Autodesk Inventor part; units mm, degrees
ref_plane "YZ Plane" through (0, 0, 0) normal (1, 0, 0) x (0, 1, 0)
ref_plane "XZ Plane" through (0, 0, 0) normal (0, 1, 0) x (-1, 0, 0)
ref_plane "XY Plane" through (0, 0, 0) normal (0, 0, 1) x (1, 0, 0)
sketch "Sketch1" plane through (0, 0, 0) normal (0, 1, 0) x (-1, 0, 0)
  line L0 (0, 0) -> (11, 0)
  line L1 (0, 0) -> (-13, 0)
  line L2 (-13, 0) -> (-13, 24)
  line L3 (-13, 24) -> (11, 24)
  line L4 (11, 24) -> (11, 0)
  circle A0 centre (-6, 17) radius 2
  circle A1 centre (-6, 7) radius 2
  circle A2 centre (-6, 17) radius 4.65
  circle A3 centre (-6, 7) radius 4.55
  dimension "d0" = 11
  dimension "d1" = 13
  dimension "d2" = 24
  dimension "d3" = 4
  dimension "d4" = 4
  dimension "d5" = 10
  dimension "d12" = 9.3
  dimension "d13" = 9.1
  dimension "d14" = 7
  dimension "d19" = 7
  dimension "d20" = 0
extrude "Extrusion1" add sketch "Sketch1" along normal blind 6 contours L1 L2 L3 L4 L0 | A2 | A3
sketch "Sketch2" plane through (0, 6, 0) normal (0, 1, 0) x (1, 0, 0)
  line L0 (-7, -15) -> (-1, -15)
  line L1 (-1, -15) -> (-1, -9)
  line L2 (-1, -9) -> (-7, -9)
  line L3 (-7, -9) -> (-7, -15)
  line L4 (13, 0) -> (-11, 0)
  line L5 (-11, -24) -> (13, -24)
  line L6 (-11, 0) -> (-11, -24)
  line L7 (-11, -24) -> (-11, 0)
  point P0 (0, 0)
  dimension "d8" = 9
  dimension "d9" = 24
extrude "Extrusion2" cut sketch "Sketch2" against normal blind 5
sketch "Sketch3" plane through (0, 6, 0) normal (0, 1, 0) x (1, 0, 0)
  circle A0 centre (6, -17) radius 2
  circle A1 centre (6, -17) radius 4.75
  circle A2 centre (6, -7) radius 4.75
  point P0 (0, 0)
  dimension "d15" = 9.5
  dimension "d16" = 9.5
extrude "Extrusion3" cut sketch "Sketch3" against normal blind 2.9
fillet "Fillet1" radius 0.2 2 edges at (1.25, 6, 17) (1.25, 6, 7)
properties part number "base"
Work out the finished part from the listing and answer in its coordinate system (mm). A direction names the side the tool comes from. Round coordinates to 2 decimals unless told otherwise and drop trailing zeros. Write each loop counter-clockwise with the first axis right and the second up, starting at its lowest first coordinate (ties: lowest second). Pieces come first, ordered by that corner, then holes. Notation, with made-up numbers: (-30.5, -21) -> (11.5, -21) arc R16 cw to (11.5, 1) -> close; hole circle Ø3 at (2, 62.25). An arc over 180 degrees is marked (long way). Write each question's results on one line, items separated by ' | '.
Q1. Section B-B, the plane y = 1.6 is taken. Write down the section's boundary in (x, z).
Data:
outline: (-11, 0) -> (13, 0) -> (13, 24) -> (-11, 24) -> close; hole (-7, 9) -> (-1, 9) -> (-1, 15) -> (-7, 15) -> close; hole circle Ø4 at (6, 7); hole circle Ø4 at (6, 17)
Q2. Flat-ended cylindrical pins translate along their axes: P1, Ø1.8, axis at x = -5, z = 13, coming from the +Y side; P2, Ø7.5, axis at x = 6, z = 17, coming from the +Y side. Find the tip coordinate at first contact, or state that the pin passes through.
Data:
P1: y = 1 | P2: y = 3.1
Q3. Section A-A, the plane x = 6 is taken. Write down the section's boundary in (y, z).
Data:
outline: (0, 0) -> (6, 0) -> (6, 2.05) arc R0.2 ccw to (5.8, 2.25) -> (3.1, 2.25) -> (3.1, 5) -> (0, 5) -> close; (0, 9) -> (3.1, 9) -> (3.1, 11.75) -> (5.8, 11.75) arc R0.2 ccw to (6, 11.95) -> (6, 12.05) arc R0.2 ccw to (5.8, 12.25) -> (3.1, 12.25) -> (3.1, 15) -> (0, 15) -> close; (0, 19) -> (3.1, 19) -> (3.1, 21.75) -> (5.8, 21.75) arc R0.2 ccw to (6, 21.95) -> (6, 24) -> (0, 24) -> close
Q4. Section D-D, the plane x = -4.75 is taken. Write down the section's boundary in (y, z), then the cut area to 3 significant figures.
Data:
outline: (0, 0) -> (6, 0) -> (6, 9) -> (1, 9) -> (1, 15) -> (6, 15) -> (6, 24) -> (0, 24) -> close | area: 114 mm^2
Q5. Determine the mould class of faces 3 (the flat face through (1, 3, 24)), 4 (the flat face through (-11, 3, 12)), 5 (the flat face through (7, 3.1, 9)) for opening direction X: released by +X, released by -X, zero draft, split by the parting line, or undercut.
Data:
face 3: zero draft | face 4: released by -X | face 5: undercut
Q6. Section C-C, the plane z = 7 is taken. Write down the section's boundary in (x, y).
Data:
outline: (-11, 0) -> (4, 0) -> (4, 3.1) -> (1.25, 3.1) -> (1.25, 5.8) arc R0.2 ccw to (1.05, 6) -> (-11, 6) -> close; (8, 0) -> (13, 0) -> (13, 6) -> (10.95, 6) arc R0.2 ccw to (10.75, 5.8) -> (10.75, 3.1) -> (8, 3.1) -> close
Q7. Which of the six approach directions +Z, -Z, +X, -X, +Y, -Y give full straight-line access (tool end or side, diameter ignored) to faces 1 (the flat face through (-4, 4, 15)), 2 (the flat face through (13, 3, 12))?
Data:
face 1: +Y | face 2: +Z, -Z, +X, +Y, -Y
Q8. Straight lines are drawn through the part: line 1 along Z through (x, y) = (6, 1.55); line 2 along Z through (x, y) = (6, 4.65); line 3 along X through (y, z) = (1.9, 9.5). For each, find the intervals that lie inside material, in ascending order. Write a range as [from, to].
Data:
line 1: [0, 5], [9, 15], [19, 24] | line 2: [0, 2.25], [11.75, 12.25], [21.75, 24] | line 3: [-11, -7], [-1, 13]
